from build123d import *

# Parameters (mm, degrees)
F0_W     = 20
F0_H     = 10
F1_DEPTH = 5
F2_W     = 5.574685
F2_H     = 2.54
F3_DEPTH = 5
F5_DEPTH = 10.001
F6_R     = 1.27
F7_DEPTH = 10.001


with BuildPart() as f1:
    # F0 (on Top) → F1 (new body)
    with BuildSketch(Plane.XY):
        with Locations((1.353551, -6.869877)):
            Rectangle(F0_W, F0_H)
    extrude(amount=F1_DEPTH)

    # F2 (on face) → F3 (join)
    with BuildSketch(Plane.XY.offset(5)):
        with Locations((-5.859107, -3.139877)):
            Rectangle(F2_W, F2_H)
        with Locations((-5.859107, -10.599877)):
            Rectangle(F2_W, F2_H)
    extrude(amount=F3_DEPTH)

    # F4 (on face) → F5 (cut, through all)
    with BuildSketch(Plane.XZ.offset(11.869877)):
        Polygon((-3.071764, 10), (-3.071764, 7.5), (-2.419111, 7.5), (-2.419111, 10.895025), (-9.260142, 10.895025), (-9.729625, 7.921636), (-8.646449, 7.5), (-8.646449, 10), align=None)
        with BuildLine():
            ThreePointArc((-8.646449, 7.5), (-5.859107, 9.988526), (-3.071764, 7.5))
            Line((-3.071764, 7.5), (-3.071764, 10))
            Line((-3.071764, 10), (-8.646449, 10))
            Line((-8.646449, 10), (-8.646449, 7.5))
        make_face()
    extrude(amount=-F5_DEPTH, mode=Mode.SUBTRACT)

    # F6 (on face) → F7 (cut, through all)
    with BuildSketch(Plane.XZ.offset(11.869877)):
        with Locations((-5.859107, 7.5)):
            Circle(F6_R)
    extrude(amount=-F7_DEPTH, mode=Mode.SUBTRACT)


solid = f1.part
The model under review builds one solid part; all positions refer to its coordinate system, in mm. A direction names the side the tool comes from. Coordinates: 2 decimals unless noted, no trailing zeros. Loops run counter-clockwise (first coordinate to the right, second up) from the corner with the lowest first, then second, coordinate; pieces in that order, holes last.
(1) Consider section A-A, the plane z = 6. Give the boundary of the cut face in (x, y), plus the area to 3 significant figures.
Determined:
outline: (-8.65, -11.87) - (-3.07, -11.87) - (-3.07, -9.33) - (-8.65, -9.33) - close; (-8.65, -4.41) - (-3.07, -4.41) - (-3.07, -1.87) - (-8.65, -1.87) - close
area: 28.3 mm2
(2) Consider section C-C, the plane x = 0.75. Give the boundary of the cut face in (y, z), plus the area to 3 significant figures.
Determined:
outline: (-11.87, 0) - (-1.87, 0) - (-1.87, 5) - (-11.87, 5) - close
area: 50.0 mm2
(3) Draft analysis for pull direction X (two halves, no side actions). For faces 1 (the flat face through (-3.072, -3, 6)), 2 (the flat face through (1, -1.87, 4)), 3 (the cylindrical face through (-5.273, -10.618, 6.373)), state which applies: +X half, -X half, draft (parallel to the pull), parting line (faces both ways), or undercut.
Determined:
face 1: +X half
face 2: draft
face 3: undercut
(4) Consider section B-B, the plane y = -10.5. Give the boundary of the cut face in (x, z), plus the area to 3 significant figures.
Determined:
outline: (-8.65, 0) - (11.35, 0) - (11.35, 5) - (-3.07, 5) - (-3.07, 7.5) arc R2.81 ccw to (-8.65, 7.5) - close; hole circle Ø2.54 at (-5.86, 7.5)
area: 119 mm2
(5) Tool access review of faces 4 (the flat face through (-8.646, -3, 6)), 5 (the flat face through (1, -11.87, 4)), 6 (the flat face through (-3.072, -11, 6)), 7 (the flat face through (-5, -4.41, 6)), 8 (the flat face through (3, -7, 5)): name each direction out of +Z, -Z, +X, -X, +Y, -Y from which nothing blocks a thin tool from reaching the whole face with its end or side.
Determined:
face 4: +Z, -Z, -X, +Y, -Y
face 5: +Z, -Z, +X, -X, -Y
face 6: +Z, +X, +Y, -Y
face 7: +Z, +X, -X
face 8: +Z, +X
(6) Wall thickness on L1, parallel to Z at x = -5.75, y = -2.25; L2, parallel to Z at x = -7.5, y = -5; L3, parallel to X at y = -3, z = 6.5: over which ranges is each line inside the solid? List them lowest first.
Determined:
L1: z = 0 to 6.23, 8.77 to 9.99
L2: z = 0 to 5
L3: x = -8.65 to -6.64, -5.08 to -3.07
(7) Insertion check: P1, Ø1, axis at y = -3.5, z = 8.5, coming from the -X side; P2, Ø1.5, axis at x = 3, y = -6.5, coming from the +Z side; P3, Ø0.8, axis at y = -10, z = 6.5, coming from the +X side. Each pin has a flat end and moves straight along its axis. Give the tip position at first contact, or say it passes through.
Determined:
P1: stops at x = -8.54
P2: stops at z = 5
P3: stops at x = -3.07
